Geometry: final body of the model. Coordinates: model frame, mm. A direction names the side the tool comes from. Round coordinates to 2 decimals unless told otherwise and drop trailing zeros. Write each loop counter-clockwise with the first axis right and the second up, starting at its lowest first coordinate (ties: lowest second). Pieces come first, ordered by that corner, then holes. Notation, with made-up numbers: M 68,84 L 111,84 A19 cw 111,119 Z; hole C -7.5,52.25 d11. An arc over 180 degrees is marked long. Answer as CSV lines item,"result". Start each with the question number.
Q1. Section query C-C on y = 23.5. Output: boundary loops of the cut face in (x, z) (3 decimals), and give its area (3 significant figures).
Q2. Section query B-B on y = 6. Output: boundary loops of the cut face in (x, z) (3 decimals), and give its area (3 significant figures).
Q3. Mould query, pull axis X, two halves, no side actions, for faces 1 (the flat face through (-66, 7, 0)), 2 (the cylindrical face through (-122.64, -1.29, -68.5)), 3 (the flat face through (0, 24, -68)). Classes: pulls with the +X half, pulls with the -X half, needs draft (parallel to the pull), parting line crosses it, or undercut.
Q4. Section query D-D on z = -53.5. Output: boundary loops of the cut face in (x, y) (3 decimals), and give its area (3 significant figures).
Q5. Reachability of faces 4 (the flat face through (-66, 8, -1.905)), 5 (the flat face through (-133.35, 24, -66)) from +Z, -Z, +X, -X, +Y, -Y: full face, straight path, thin tool, end or side. Return the list, or none.
Q6. Ray query, probe 1 along X at (y, z) = (38, -26) (3 decimals); probe 2 along Y at (x, z) = (-37, -87). Return the intervals inside material, ascending.
Q7. First-contact query: pin 1 (6 mm diameter, centred on x = -122.555, z = -66.675, fed in from +Y); pin 2 (4 mm diameter, centred on y = 13.5, z = -76, fed in from +X); pin 3 (3 mm diameter, centred on x = -85.5, y = 32.5, fed in from +Z) (3 decimals). Flat tips, straight axial feed; report the tip coordinate or a pass-through.
Q8. Section query A-A on x = -100. Output: boundary loops of the cut face in (y, z) (3 decimals).
Autodesk Inventor part; units mm, degrees
ref_plane "YZ Plane" through (0, 0, 0) normal (1, 0, 0) x (0, 1, 0)
ref_plane "XZ Plane" through (0, 0, 0) normal (0, 1, 0) x (-1, 0, 0)
ref_plane "XY Plane" through (0, 0, 0) normal (0, 0, 1) x (1, 0, 0)
sketch "Sketch1" plane through (0, 0, 0) normal (0, 1, 0) x (-1, 0, 0)
  line L0 (0, 0) -> (133.35, 0)
  line L1 (133.35, 0) -> (133.35, -133.35)
  line L2 (133.35, -133.35) -> (0, -133.35)
  line L3 (0, -133.35) -> (0, 0)
  line L4 (131.445, -131.445) -> (1.905, -131.445)
  line L5 (1.905, -131.445) -> (1.905, -1.905)
  line L6 (1.905, -1.905) -> (131.445, -1.905)
  line L7 (131.445, -1.905) -> (131.445, -131.445)
  line L8 (131.445, -131.445) -> (1.905, -1.905) construction
  line L9 (1.905, -131.445) -> (131.445, -1.905) construction
  point P0 (66.675, -66.675)
  dimension "d0" = 133.35
  dimension "d1" = 133.35
  dimension "d2" = 129.54
  dimension "d3" = 129.54
extrude "Extrusion1" add sketch "Sketch1" along normal blind 50.8
extrude "Extrusion2" add sketch "Sketch1" against normal blind 2.54 contours L0 L1 L2 L3 | L4 L5 L6 L7
fillet "Fillet1" radius 1.27 8 edges at (0, 24.13, 0) (0, -2.54, -66.675) (-66.675, -2.54, 0) (0, 24.13, -133.35) (-66.675, -2.54, -133.35) (-133.35, 24.13, -133.35) (-133.35, -2.54, -66.675) (-133.35, 24.13, 0)
sketch "Sketch2" plane through (0, 0, 0) normal (0, 1, 0) x (1, 0, 0)
  line L0 (-131.445, 1.905) -> (-131.445, 131.445)
  line L1 (-1.905, 1.905) -> (-131.445, 1.905)
  line L2 (-1.905, 131.445) -> (-1.905, 1.905)
  line L3 (-131.445, 131.445) -> (-1.905, 131.445)
  line L4 (-66.675, 66.675) -> (-10.795, 66.675)
  line L5 (-66.675, 66.675) -> (-10.795, 66.675) construction
  line L6 (-10.795, 66.675) -> (-122.555, 66.675)
  point P0 (0, 0)
  dimension "d9" = 55.88
  dimension "d10" = 0
  dimension "d11" = 111.76
hole "Hole1" at (-10.795, 0, -66.675) at (-122.555, 0, -66.675) direction (0, -1, 0) diameter 3.6576 end through all
sketch "Sketch3" plane through (-132.08, -1.27, 0) normal (0, 0, 1) x (1, 0, 0)
  line L0 (130.175, 1.27) -> (0.635, 1.27)
  line L1 (65.405, 1.27) -> (65.405, 13.97)
  line L2 (65.405, 13.97) -> (109.855, 13.97)
  line L3 (109.855, 13.97) -> (20.955, 13.97)
  line L4 (20.955, 13.97) -> (20.955, 39.37)
  line L5 (20.955, 39.37) -> (109.855, 39.37)
  line L6 (109.855, 39.37) -> (109.855, 13.97)
  point P0 (132.08, 1.27)
  dimension "d19" = 12.7
  dimension "d20" = 44.45
  dimension "d21" = 88.9
  dimension "d22" = 25.4
extrude "Extrusion3" cut sketch "Sketch3" against normal blind 2.54
properties part number "TC720 box"
Entries:
1,outline,"M -133.35,-132.08 A1.27 ccw -132.08,-133.35 L -1.27,-133.35 A1.27 ccw 0,-132.08 L 0,-1.27 A1.27 ccw -1.27,0 L -22.225,0 L -22.225,-1.905 L -1.905,-1.905 L -1.905,-131.445 L -131.445,-131.445 L -131.445,-1.905 L -111.125,-1.905 L -111.125,0 L -132.08,0 A1.27 ccw -133.35,-1.27 Z"
1,area,"831 mm^2"
2,outline,"M -133.35,-132.08 A1.27 ccw -132.08,-133.35 L -1.27,-133.35 A1.27 ccw 0,-132.08 L 0,-1.27 A1.27 ccw -1.27,0 L -132.08,0 A1.27 ccw -133.35,-1.27 Z; hole M -131.445,-131.445 L -1.905,-131.445 L -1.905,-1.905 L -131.445,-1.905 Z"
2,area,"1,000 mm^2"
3,face 1,"needs draft"
3,face 2,"undercut"
3,face 3,"pulls with the +X half"
4,outline,"M -133.35,-1.27 A1.27 ccw -132.08,-2.54 L -1.27,-2.54 A1.27 ccw 0,-1.27 L 0,50.8 L -1.905,50.8 L -1.905,0 L -131.445,0 L -131.445,50.8 L -133.35,50.8 Z"
4,area,"532 mm^2"
5,face 4,"+Y"
5,face 5,"+Z, -Z, -X, +Y, -Y"
6,probe 1,"x = -133.35 to -131.445, -1.905 to 0"
6,probe 2,"y = -2.54 to 0"
7,pin 1,"stops at y = 0"
7,pin 2,"stops at x = 0"
7,pin 3,"stops at z = -131.445"
8,outline,"M -2.54,-132.08 A1.27 ccw -1.27,-133.35 L 50.8,-133.35 L 50.8,-131.445 L 0,-131.445 L 0,-1.905 L 12.7,-1.905 L 12.7,0 L -1.27,0 A1.27 ccw -2.54,-1.27 Z; M 38.1,-1.905 L 50.8,-1.905 L 50.8,0 L 38.1,0 Z"
